```python
from build123d import *

# Parameters (mm, degrees)
EXTRUDE_1_DEPTH = 5
FILLET_1_R      = 20


with BuildPart() as part:
    # 草图1 → 凸台-拉伸1 (new body)
    with BuildSketch(Plane.XY):
        Polygon((-101, 0), (-80.5, 0), (-80.5, 7), (-82, 7), (-82, 9.9), (-80.5, 9.9), (-80.5, 11), (-76.5, 11), (-76.5, 9.9), (-75, 9.9), (-75, 7), (-76.5, 7), (-76.5, 0), (-70.5, 0), (-70.5, -5), (-40.5, -5), (-40.5, 0), (-34.5, 0), (-34.5, 7), (-36, 7), (-36, 9.9), (-34.5, 9.9), (-34.5, 11), (-30.5, 11), (-30.5, 9.9), (-29, 9.9), (-29, 7), (-30.5, 7), (-30.5, 0), (0, 0), (0, 25), (-5, 25), (-5, 18), (-10, 18), (-10, 25), (-111, 25), (-111, 0), (-106, 0), (-106, 5.5), (-101, 5.5), align=None)
    extrude(amount=EXTRUDE_1_DEPTH)

    # 圆角1
    fillet_1_edges = [part.edges().sort_by_distance(p)[0] for p in [
        (-111, 25, 2.5),
    ]]
    fillet(fillet_1_edges, radius=FILLET_1_R)


solid = part.part
```
Could you check a few things on this model? Use its own coordinates, in mm. A direction names the side the tool comes from. Round coordinates to 2 decimals unless told otherwise and drop trailing zeros. Write each loop counter-clockwise with the first axis right and the second up, starting at its lowest first coordinate (ties: lowest second). Pieces come first, ordered by that corner, then holes. Notation, with made-up numbers: M 75,-8 L 81,-8 A24 cw 81,30 Z; hole C -10,-16 d10. An arc over 180 degrees is marked long. Answer in a Markdown table with one row per item. Add a question column.
Q1. Imagine slicing it at B-B (y = 20). Please give me the cut outline in (x, z).
Q2. Imagine slicing it at A-A (y = 1.5). Please give me the cut outline in (x, z), then the cut area to 3 significant figures.
Q3. On a 3-axis mill with a long thin cutter (end or side, diameter ignored), from which of +Z, -Z, +X, -X, +Y, -Y can I reach the whole of each face in a straight line? I mean faces 1 (the flat face through (-36, 8, 2)), 2 (the flat face through (-10, 21, 2)), 3 (the flat face through (-33, 11, 2)), 4 (the flat face through (-15, 0, 2)). Say none if no direction works.
Q4. Will these pins go through, and if not, where does the flat tip stop? pin 1 Ø0.5 at (y, z) = (10.5, 3) entering from -X; pin 2 Ø1.5 at (x, z) = (-109.5, 1.5) entering from -Y; pin 3 Ø2.5 at (y, z) = (8, 2) entering from -X.
Q5. If I drill on line 1 (X direction, y = 2.5, z = 3); line 2 (X direction, y = 8, z = 0.8); line 3 (X direction, y = 9.5, z = 0.5), over which ranges is the centre line in solid material (lowest first)? Write a range as from..to.
Q6. Imagine slicing it at C-C (x = -39.5). Please give me the cut outline in (y, z).
Q7. If we mould it in two halves opening along X, with no side actions, what happens to faces 5 (the flat face through (-91, 0, 2)), 6 (the flat face through (-82, 8, 2)), 7 (the flat face through (0, 12, 2))? For each: +X half, -X half, draft (parallel to the pull), parting line (faces both ways), or undercut.
Values:
| question | item | result |
|---|---|---|
| 1 | outline | M -104.23,0 L -10,0 L -10,5 L -104.23,5 Z; M -5,0 L 0,0 L 0,5 L -5,5 Z |
| 2 | outline | M -111,0 L -106,0 L -106,5 L -111,5 Z; M -101,0 L -80.5,0 L -80.5,5 L -101,5 Z; M -76.5,0 L -34.5,0 L -34.5,5 L -76.5,5 Z; M -30.5,0 L 0,0 L 0,5 L -30.5,5 Z |
| 2 | area | 490 mm^2 |
| 3 | face 1 | +Z, -Z |
| 3 | face 2 | +Z, -Z, +Y |
| 3 | face 3 | +Z, -Z, -Y |
| 3 | face 4 | +Z, -Z, +X, -Y |
| 4 | pin 1 | x = -110.3 |
| 4 | pin 2 | y = 0 |
| 4 | pin 3 | x = -110.92 |
| 5 | line 1 | -111..-106, -101..-80.5, -76.5..-34.5, -30.5..0 |
| 5 | line 2 | -110.77..-82, -75..-36, -29..0 |
| 5 | line 3 | -110.49..-82, -75..-36, -29..0 |
| 6 | outline | M 0,0 L 25,0 L 25,5 L 0,5 Z |
| 7 | face 5 | draft |
| 7 | face 6 | undercut |
| 7 | face 7 | +X half |
